Geometry: final body of the model. Coordinates: model frame, mm. A direction names the side the tool comes from. Give positions to 0.01 mm unless a question says otherwise; leave off trailing zeros. Write each loop counter-clockwise with the first axis right and the second up, starting at its lowest first coordinate (ties: lowest second). Pieces come first, ordered by that corner, then holes.
from build123d import *

# Parameters (mm, degrees)
BOSS_EXTRUDE1_DEPTH = 60
SKETCH6_W           = 76.2
SKETCH6_H           = 139.7
BOSS_EXTRUDE3_DEPTH = 3
SKETCH7_W           = 254.695348458
SKETCH7_H           = 135.329086622
CUT_EXTRUDE1_DEPTH  = 76.2
SKETCH8_W           = 10
SKETCH8_H           = 5
CUT_EXTRUDE2_DEPTH  = 172.74190537
SKETCH9_W           = 55
SKETCH9_H           = 40
CUT_EXTRUDE3_DEPTH  = 246.885251985
SKETCH10_W          = 200.764393162
SKETCH10_H          = 14.388440844
CUT_EXTRUDE4_DEPTH  = 15
BOSS_EXTRUDE4_DEPTH = 4
BOSS_EXTRUDE5_DEPTH = 4
SKETCH13_W          = 181.59007752
SKETCH13_H          = 354.992238287
CUT_EXTRUDE5_DEPTH  = 101.75


with BuildPart() as part:
    # Sketch1 → Boss-Extrude1 (new body)
    with BuildSketch(Plane.XY):
        with BuildLine():
            Line((-101.6, 101.6), (-101.6, -38.1))
            ThreePointArc((-101.6, -38.1), (-83.001280605, -83.001280605), (-38.1, -101.6))
            Line((-38.1, -101.6), (38.1, -101.6))
            ThreePointArc((38.1, -101.6), (83.001280605, -83.001280605), (101.6, -38.1))
            Line((101.6, -38.1), (101.6, 101.6))
            Line((101.6, 101.6), (-101.6, 101.6))
        make_face()
        with BuildLine():
            Line((-98.6, 98.6), (-98.6, -38.1))
            ThreePointArc((-98.6, -38.1), (-80.879960262, -80.879960262), (-38.1, -98.6))
            Line((-38.1, -98.6), (38.1, -98.6))
            ThreePointArc((38.1, -98.6), (80.879960262, -80.879960262), (98.6, -38.1))
            Line((98.6, -38.1), (98.6, 98.6))
            Line((98.6, 98.6), (-98.6, 98.6))
        make_face(mode=Mode.SUBTRACT)
    extrude(amount=BOSS_EXTRUDE1_DEPTH)

    # Sweep2: sweep along a path in Sketch5
    with BuildLine(Plane.XY.offset(60)) as sweep2_path:
        Line((-100.1, 101.6), (-100.1, -38.1))
        ThreePointArc((-100.1, -38.1), (-81.940620434, -81.940620434), (-38.1, -100.1))
        Line((-38.1, -100.1), (38.1, -100.1))
        ThreePointArc((38.1, -100.1), (81.940620434, -81.940620434), (100.1, -38.1))
        Line((100.1, -38.1), (100.1, 101.6))
    # Sketch3 → Sweep2 (sweep)
    with BuildSketch(Plane(origin=(0, 101.6, 0), x_dir=(1, 0, 0), z_dir=(0, 1, 0))):
        with BuildLine():
            Line((-38.1, -91.039099262), (-88.9, -91.039099262))
            ThreePointArc((-88.9, -91.039099262), (-95.981959893, -87.480761361), (-98.6, -80))
            Line((-98.6, -80), (-98.6, -60))
            Line((-98.6, -60), (-101.6, -60))
            Line((-101.6, -60), (-101.6, -80))
            ThreePointArc((-101.6, -80), (-98.157592659, -89.649805752), (-88.9, -94.039099262))
            Line((-88.9, -94.039099262), (-38.1, -94.039099262))
            Line((-38.1, -94.039099262), (-38.1, -91.039099262))
        make_face()
    sweep(path=sweep2_path.line)

    # Sketch6 → Boss-Extrude3 (add)
    with BuildSketch(Plane.XY.offset(94.039099262)):
        with Locations((0, 31.75)):
            Rectangle(SKETCH6_W, SKETCH6_H)
    extrude(amount=-BOSS_EXTRUDE3_DEPTH)

    # Sketch7 → Cut-Extrude1 (cut)
    with BuildSketch(Plane(origin=(0, 101.6, 0), x_dir=(1, 0, 0), z_dir=(0, 1, 0))):
        with Locations((-4.889183354, -23.374555951)):
            Rectangle(SKETCH7_W, SKETCH7_H)
    extrude(amount=-CUT_EXTRUDE1_DEPTH, mode=Mode.SUBTRACT)

    # Sketch8 → Cut-Extrude2 (cut, through all)
    with BuildSketch(Plane.XY.offset(94.039099262)):
        with Locations((0, 39.440517612)):
            Rectangle(SKETCH8_W, SKETCH8_H)
    extrude(amount=-CUT_EXTRUDE2_DEPTH, mode=Mode.SUBTRACT)

    # Sketch9 → Cut-Extrude3 (cut, through all)
    with BuildSketch(Plane(origin=(0, -101.6, 0), x_dir=(-1, 0, 0), z_dir=(0, -1, 0))):
        with Locations((0, -20)):
            Rectangle(SKETCH9_W, SKETCH9_H)
    extrude(amount=-CUT_EXTRUDE3_DEPTH, mode=Mode.SUBTRACT)

    # Sketch10 → Cut-Extrude4 (cut)
    with BuildSketch(Plane(origin=(0, 101.6, 0), x_dir=(1, 0, 0), z_dir=(0, 1, 0))):
        with Locations((0, -94.039099262)):
            Rectangle(SKETCH10_W, SKETCH10_H)
    extrude(amount=-CUT_EXTRUDE4_DEPTH, mode=Mode.SUBTRACT)

    # Sketch11 → Boss-Extrude4 (add)
    with BuildSketch(Plane(origin=(0, -98.6, 0), x_dir=(1, 0, 0), z_dir=(0, 1, 0))):
        Polygon((0, -80), (1.5, -80), (1.5, -40), (0, -40), (-1.5, -40), (-1.5, -80), align=None)
    extrude(amount=BOSS_EXTRUDE4_DEPTH)

    # Sketch12 → Boss-Extrude5 (add)
    with BuildSketch(Plane(origin=(0, 0, 91.039099262), x_dir=(-1, 0, 0), z_dir=(0, 0, -1))):
        Polygon((-1.5, -88.9), (0, -88.9), (1.5, -88.9), (1.5, 36.940517612), (-1.5, 36.940517612), align=None)
    extrude(amount=BOSS_EXTRUDE5_DEPTH)

    # Sketch13 → Cut-Extrude5 (cut)
    with BuildSketch(Plane(origin=(101.6, 0, 0), x_dir=(0, 0, -1), z_dir=(1, 0, 0))):
        with Locations((-39.565471337, -8.440264941)):
            Rectangle(SKETCH13_W, SKETCH13_H)
    extrude(amount=-CUT_EXTRUDE5_DEPTH, mode=Mode.SUBTRACT)


with BuildPart() as cut_extrude5_kept_piece:
    # of the separate pieces the step leaves, the one the design keeps (cut_extrude5_pieces_kept)
    add(part.part.solids().sort_by_distance((-101.6, 25.4, 0))[0])


solid = cut_extrude5_kept_piece.part
Q1. Section A-A on z = 48.5. Output: boundary loops of the cut face in (x, y), plus the area to 3 significant figures.
Filled sheet:
outline: (-101.6, -38.1) arc R63.5 ccw to (-38.1, -101.6) - (-0.15, -101.6) - (-0.15, -94.6) - (-1.5, -94.6) - (-1.5, -98.6) - (-38.1, -98.6) arc R60.5 cw to (-98.6, -38.1) - (-98.6, 25.4) - (-101.6, 25.4) - close
area: 602 mm2
Q2. Access query for faces 4 (the flat face through (-0.15, -42.3, 87.2)), 5 (the flat face through (-14, -100, 40)), 6 (the flat face through (-49, 0, 91.039)), 7 (the flat face through (-24, -101.6, 48)), 8 (the flat face through (-2, 36.941, 92)). Directions: +Z, -Z, +X, -X, +Y, -Y. A direction counts if a zero-diameter tool reaches every point of the face in a straight line with its end or side. Return the directions, or none.
Filled sheet:
face 4: +Z, -Z, +X, +Y, -Y
face 5: -Z, +X, +Y, -Y
face 6: -Z, +Y
face 7: +Z, -Z, +X, -X, -Y
face 8: +Z, -Z, +X
Q3. Pin query (flat end, axial travel): P1, Ø0.9, axis at x = -3, z = 92.5, coming from the -Y side; P2, Ø4, axis at y = -40, z = 9.5, coming from the +X side; P3, Ø1.5, axis at x = -52.5, z = 50, coming from the -Y side. Return the tip coordinate at first contact, or that it passes through.
Filled sheet:
P1: stops at y = -95.28
P2: stops at x = -98.47
P3: stops at y = -100.12
Q4. Section D-D on z = 22.5. Output: boundary loops of the cut face in (x, y), plus the area to 3 significant figures.
Filled sheet:
outline: (-101.6, -38.1) arc R63.5 ccw to (-38.1, -101.6) - (-27.5, -101.6) - (-27.5, -98.6) - (-38.1, -98.6) arc R60.5 cw to (-98.6, -38.1) - (-98.6, 25.4) - (-101.6, 25.4) - close
area: 514 mm2
Q5. Pull-direction query (X, two-part tool) for faces 1 (the flat face through (-98.6, -7, 41)), 2 (the flat face through (-45, 0, 94.039)), 3 (the flat face through (-1.5, -27, 89)); classes: released by +X, released by -X, zero draft, split by the parting line, or undercut.
Filled sheet:
face 1: released by +X
face 2: zero draft
face 3: undercut
Q6. Section B-B on y = -22. Output: boundary loops of the cut face in (x, z), plus the area to 3 significant figures.
Filled sheet:
outline: (-101.6, 0) - (-98.6, 0) - (-98.6, 80) arc R10.57 cw to (-88.9, 91.04) - (-1.5, 91.04) - (-1.5, 87.04) - (-0.15, 87.04) - (-0.15, 94.04) - (-88.9, 94.04) arc R13.39 ccw to (-101.6, 80) - close
area: 568 mm2
Q7. Section C-C on x = -8.5. Output: boundary loops of the cut face in (y, z).
Filled sheet:
outline: (-101.6, 40) - (-98.6, 40) - (-98.6, 80) arc R10.57 cw to (-88.9, 91.04) - (86.6, 91.04) - (86.6, 94.04) - (-88.9, 94.04) arc R13.39 ccw to (-101.6, 80) - close
Q8. Ray query, line 1 along X through (y, z) = (-20, 47); line 2 along Z through (x, y) = (-13, 30). Return the intervals inside material, ascending.
Filled sheet:
line 1: x = -101.6 to -98.6
line 2: z = 91.04 to 94.04
